The model under review builds one solid part; all positions refer to its coordinate system, in mm. A direction names the side the tool comes from. Coordinates: 2 decimals unless noted, no trailing zeros. Order: outer loops, then holes, each group sorted by start corner. A loop starts at its lowest first (then second) coordinate and runs counter-clockwise, first axis right, second up. Notation, with made-up numbers: (80, -25.5) - (117, -25.5) arc R21 cw to (117, -8.5) - close; hole circle Ø7 at (42.5, 49). An arc over 180 degrees is marked (long way). Answer in a Markdown table with one row per item.
```python
from build123d import *

# Parameters (mm, degrees)
SKETCH_1_R          = 2.5
EXTRUDE_1_DEPTH     = 10
SKETCH_2_R          = 2
CUT_EXTRUDE_1_DEPTH = 15
SKETCH_3_R          = 2
CUT_EXTRUDE_2_DEPTH = 15


with BuildPart() as part:
    # ｽｹｯﾁ1 → ﾎﾞｽ - 押し出し1 (new body)
    with BuildSketch(Plane.XY):
        with BuildLine():
            ThreePointArc((5.736159103, 27.814680993), (0, 28.4), (-5.736159103, 27.814680993))
            Line((-5.736159103, 27.814680993), (-26.95629989, -8.939680993))
            ThreePointArc((-26.95629989, -8.939680993), (-24.595121467, -14.2), (-21.220140787, -18.875))
            Line((-21.220140787, -18.875), (21.220140787, -18.875))
            ThreePointArc((21.220140787, -18.875), (24.595121467, -14.2), (26.95629989, -8.939680993))
            Line((26.95629989, -8.939680993), (5.736159103, 27.814680993))
        make_face()
        with Locations((-20.56810334, -11.875)):
            Circle(SKETCH_1_R, mode=Mode.SUBTRACT)
        with Locations((20.56810334, -11.875)):
            Circle(SKETCH_1_R, mode=Mode.SUBTRACT)
        with BuildLine():
            ThreePointArc((6, 0), (-5.449489743, -2.51058988), (3.898979486, 4.560477932))
            Line((3.898979486, 4.560477932), (5.408587988, 5.432050808))
            Line((5.408587988, 5.432050808), (7.408587988, 1.967949192))
            Line((7.408587988, 1.967949192), (5.898979486, 1.096376317))
            ThreePointArc((5.898979486, 1.096376317), (5.974691495, 0.550510257), (6, 0))
        make_face(mode=Mode.SUBTRACT)
        with Locations((0, 23.75)):
            Circle(SKETCH_1_R, mode=Mode.SUBTRACT)
    extrude(amount=EXTRUDE_1_DEPTH)

    # ｽｹｯﾁ2 → ｶｯﾄ - 押し出し1 (cut)
    with BuildSketch(Plane(origin=(16.346229496, 9.4375, 0), x_dir=(0, 0, -1), z_dir=(0.8660254037844386, 0.5, 0))):
        with Locations(Location((-5, 0, 0), (0, 0, 90))):
            Circle(SKETCH_2_R)
    extrude(amount=-CUT_EXTRUDE_1_DEPTH, mode=Mode.SUBTRACT)

    # ｽｹｯﾁ3 → ｶｯﾄ - 押し出し2 (cut)
    with BuildSketch(Plane.XZ.offset(18.875)):
        with Locations((0, 5)):
            Circle(SKETCH_3_R)
    extrude(amount=-CUT_EXTRUDE_2_DEPTH, mode=Mode.SUBTRACT)


solid = part.part
```
Item 1: We need section A-A, the plane x = 0. Write out the cut boundary in (y, z) (3 decimals), then the cut area to 3 significant figures.
Check values:
| item | result |
|---|---|
| outline | (-18.875, 0) - (-6, 0) - (-6, 3) - (-18.875, 3) - close; (-18.875, 7) - (-6, 7) - (-6, 10) - (-18.875, 10) - close; (6, 0) - (21.25, 0) - (21.25, 10) - (6, 10) - close; (26.25, 0) - (28.4, 0) - (28.4, 10) - (26.25, 10) - close |
| area | 251 mm^2 |
Item 2: We need section B-B, the plane y = -12.5. Write out the cut boundary in (x, z).
Check values:
| item | result |
|---|---|
| outline | (-25.5, 0) - (-22.99, 0) - (-22.99, 10) - (-25.5, 10) - close; (-18.15, 0) - (18.15, 0) - (18.15, 10) - (-18.15, 10) - close; (22.99, 0) - (25.5, 0) - (25.5, 10) - (22.99, 10) - close; hole circle Ø4 at (0, 5) |
Item 3: We need section D-D, the plane y = -2. Write out the cut boundary in (x, z).
Check values:
| item | result |
|---|---|
| outline | (-22.95, 0) - (-5.66, 0) - (-5.66, 10) - (-22.95, 10) - close; (5.66, 0) - (22.95, 0) - (22.95, 10) - (5.66, 10) - close |
Item 4: Tool access review of faces 4 (the face through (0, -12, 7)), 5 (the face through (6.664, 1.538, 4.93)), 6 (the face through (10.909, 7.54, 6.686)): name each direction out of +Z, -Z, +X, -X, +Y, -Y from which nothing blocks a thin tool from reaching the whole face with its end or side.
Check values:
| item | result |
|---|---|
| face 4 | -Y |
| face 5 | +Z, -Z |
| face 6 | none |
Item 5: Mouldability with a two-part tool opening along X and no side actions: class faces 1 (the face through (-0.33, 26.23, 4.93)), 2 (the face through (-0.3, -18.875, 2.7)), 3 (the face through (0.1, 28.4, 4.9)) as +X half, -X half, draft (parallel to the pull), parting line (faces both ways), or undercut.
Check values:
| item | result |
|---|---|
| face 1 | undercut |
| face 2 | draft |
| face 3 | parting line |
Item 6: To check wall thickness, follow line 1 (Y direction, x = 0, z = 2.75) (3 decimals); line 2 (Y direction, x = 0, z = 4.25); line 3 (Z direction, x = 0, y = -15.5). State the ranges of each line that lie inside material, in increasing order. Write a range as from..to.
Check values:
| item | result |
|---|---|
| line 1 | -18.875..-6, 6..21.25, 26.25..28.4 |
| line 2 | 6..21.25, 26.25..28.4 |
| line 3 | 0..3, 7..10 |
Item 7: Clearance check with flat-ended pins moving along their axes: pin 1 Ø9.5 at (x, y) = (0, 0) entering from +Z; pin 2 Ø4 at (y, z) = (20.5, 1.5) entering from +X; pin 3 Ø6 at (y, z) = (-0.5, 9) entering from -X. State where each tip first meets the part, or that it passes through.
Check values:
| item | result |
|---|---|
| pin 1 | through |
| pin 2 | x = 11.11 |
| pin 3 | x = -23.82 |
Item 8: We need section C-C, the plane y = 25. Write out the cut boundary in (x, z), then the cut area to 3 significant figures.
Check values:
| item | result |
|---|---|
| outline | (-7.36, 0) - (-2.17, 0) - (-2.17, 10) - (-7.36, 10) - close; (2.17, 0) - (7.36, 0) - (7.36, 10) - (2.17, 10) - close |
| area | 104 mm^2 |
